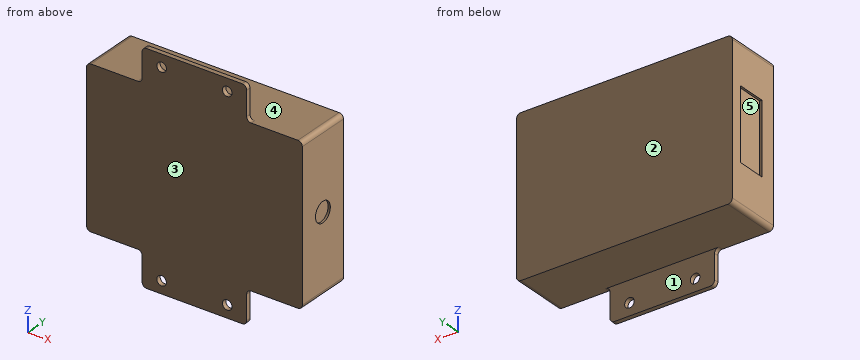
from build123d import *

# Parameters (mm, degrees)
SKETCH1_W            = 97
SKETCH1_H            = 100
BOSS_EXTRUDE1_DEPTH  = 25
M4_CLEARANCE_HOLE1_D = 4.3
SKETCH5_W            = 32
SKETCH5_H            = 13
CUT_EXTRUDE1_DEPTH   = 1
SKETCH6_R            = 4.5
CUT_EXTRUDE2_DEPTH   = 1
SKETCH7_W            = 97
SKETCH7_H            = 15
CUT_EXTRUDE3_DEPTH   = 23
SKETCH8_W            = 25
SKETCH8_H            = 15
CUT_EXTRUDE4_DEPTH   = 74.357003756
FILLET1_R            = 2


with BuildPart() as part:
    # Sketch1 → Boss-Extrude1 (new body)
    with BuildSketch(Plane(origin=(0, 0, 0), x_dir=(1, 0, 0), z_dir=(0, 1, 0))):
        Rectangle(SKETCH1_W, SKETCH1_H)
    extrude(amount=BOSS_EXTRUDE1_DEPTH)

    # M4 Clearance Hole1 (through all)
    with Locations(Plane(origin=(0, 25, 0), x_dir=(1, 0, 0), z_dir=(0, 1, 0))):
        with Locations((-14.75, 44.5), (14.75, 44.5), (-14.75, -44.5), (14.75, -44.5)):
            Hole(M4_CLEARANCE_HOLE1_D / 2)

    # Sketch5 → Cut-Extrude1 (cut)
    with BuildSketch(Plane.ZY.offset(48.5)):
        with Locations((0, 13.5)):
            Rectangle(SKETCH5_W, SKETCH5_H)
    extrude(amount=-CUT_EXTRUDE1_DEPTH, mode=Mode.SUBTRACT)

    # Sketch6 → Cut-Extrude2 (cut)
    with BuildSketch(Plane(origin=(48.5, 0, 0), x_dir=(0, 0, -1), z_dir=(1, 0, 0))):
        with Locations((0, 12.5)):
            Circle(SKETCH6_R)
    extrude(amount=-CUT_EXTRUDE2_DEPTH, mode=Mode.SUBTRACT)

    # Sketch7 → Cut-Extrude3 (cut)
    with BuildSketch(Plane(origin=(0, 25, 0), x_dir=(1, 0, 0), z_dir=(0, 1, 0))):
        with Locations((0, 42.5)):
            Rectangle(SKETCH7_W, SKETCH7_H)
        with Locations((0, -42.5)):
            Rectangle(SKETCH7_W, SKETCH7_H)
    extrude(amount=-CUT_EXTRUDE3_DEPTH, mode=Mode.SUBTRACT)

    # Sketch8 → Cut-Extrude4 (cut, through all)
    with BuildSketch(Plane(origin=(0, 2, 0), x_dir=(1, 0, 0), z_dir=(0, 1, 0))):
        with Locations((-36, 42.5)):
            Rectangle(SKETCH8_W, SKETCH8_H)
        with Locations((36, 42.5)):
            Rectangle(SKETCH8_W, SKETCH8_H)
        with Locations((-36, -42.5)):
            Rectangle(SKETCH8_W, SKETCH8_H)
        with Locations((36, -42.5)):
            Rectangle(SKETCH8_W, SKETCH8_H)
    extrude(amount=-CUT_EXTRUDE4_DEPTH, mode=Mode.SUBTRACT)

    # Fillet1
    fillet1_edges = [part.edges().sort_by_distance(p)[0] for p in [
        (23.5, 1, -35),
        (23.5, 1, -50),
        (-23.5, 1, 35),
        (-23.5, 1, 50),
        (23.5, 1, 50),
        (23.5, 1, 35),
        (-23.5, 1, -50),
        (-23.5, 1, -35),
        (48.5, 12.5, -35),
        (-48.5, 12.5, -35),
        (48.5, 12.5, 35),
        (-48.5, 12.5, 35),
    ]]
    fillet(fillet1_edges, radius=FILLET1_R)


solid = part.part
Design review of the part built by this model. Coordinates are the model's own, in mm. Face numbers are marked on the shaded views. A direction names the side the tool comes from. Give positions to 0.01 mm unless a question says otherwise; leave off trailing zeros. Loops run counter-clockwise (first coordinate to the right, second up) from the corner with the lowest first, then second, coordinate; pieces in that order, holes last. Notation, with made-up numbers: (-20, 48.5) -> (23, 48.5) arc R17 ccw to (23, 52.5) -> close; hole circle Ø5 at (54, -10.5). An arc over 180 degrees is marked (long way). One line per question, with ' | ' between items. Start each with the question number.
(1) We need section A-A (z = -44.5). State the section outline as (x, y) points, and give its area (3 significant figures).
(2) We need section D-D (x = -5.5). State the section outline as (y, z) points.
(3) Draft analysis for pull direction Y (two halves, no side actions). For the marked faces 3, 4 and 5, state which applies: +Y half, -Y half, draft (parallel to the pull), parting line (faces both ways), or undercut.
(4) Insertion check: P1, Ø1.1, axis at x = -48, z = 7.5, coming from the -Y side; P2, Ø2, axis at y = 1, z = -44.5, coming from the -X side; P3, Ø5, axis at x = -6, y = 5.5, coming from the +Z side; P4, Ø12, axis at x = -9.5, z = 45.5, coming from the +Y side. Each pin has a flat end and moves straight along its axis. Give the tip position at first contact, or say it passes through.
(5) For the marked faces 1 and 2, list the 3-axis set-ups (+Z, -Z, +X, -X, +Y, -Y) from which the entire face can be reached by the end or side of a thin tool; tool diameter is ignored.
(6) For line 1 (Z direction, x = 14.75, y = 0.7); line 2 (X direction, y = 0.8, z = -44.5); line 3 (Z direction, x = 30, y = 18.75), list the stretches that pass through material, from the lowest coordinate up.
(7) We need section B-B (x = 14.75). State the section outline as (y, z) points, and give its area (3 significant figures).
(8) We need section C-C (y = 18.5). State the section outline as (x, z) points.
The answers:
1) outline: (-23.5, 0) -> (-16.9, 0) -> (-16.9, 2) -> (-23.5, 2) -> close; (-12.6, 0) -> (12.6, 0) -> (12.6, 2) -> (-12.6, 2) -> close; (16.9, 0) -> (23.5, 0) -> (23.5, 2) -> (16.9, 2) -> close | area: 76.8 mm^2
2) outline: (0, -50) -> (2, -50) -> (2, -35) -> (25, -35) -> (25, 35) -> (2, 35) -> (2, 50) -> (0, 50) -> close
3) face 3: -Y half | face 4: draft | face 5: undercut
4) P1: stops at y = 0 | P2: stops at x = -23.5 | P3: stops at z = 35 | P4: stops at y = 2
5) face 1: -Z, +X, -X, +Y | face 2: +Z, -Z, +X, -X, +Y
6) line 1: z = -50 to -46.65, -42.35 to 42.35, 46.65 to 50 | line 2: x = -23.5 to -16.9, -12.6 to 12.6, 16.9 to 23.5 | line 3: z = -35 to 35
7) outline: (0, -50) -> (2, -50) -> (2, -46.65) -> (0, -46.65) -> close; (0, -42.35) -> (2, -42.35) -> (2, -35) -> (25, -35) -> (25, 35) -> (2, 35) -> (2, 42.35) -> (0, 42.35) -> close; (0, 46.65) -> (2, 46.65) -> (2, 50) -> (0, 50) -> close | area: 1,790 mm^2
8) outline: (-48.5, -33) arc R2 ccw to (-46.5, -35) -> (46.5, -35) arc R2 ccw to (48.5, -33) -> (48.5, 33) arc R2 ccw to (46.5, 35) -> (-46.5, 35) arc R2 ccw to (-48.5, 33) -> (-48.5, 16) -> (-47.5, 16) -> (-47.5, -16) -> (-48.5, -16) -> close
